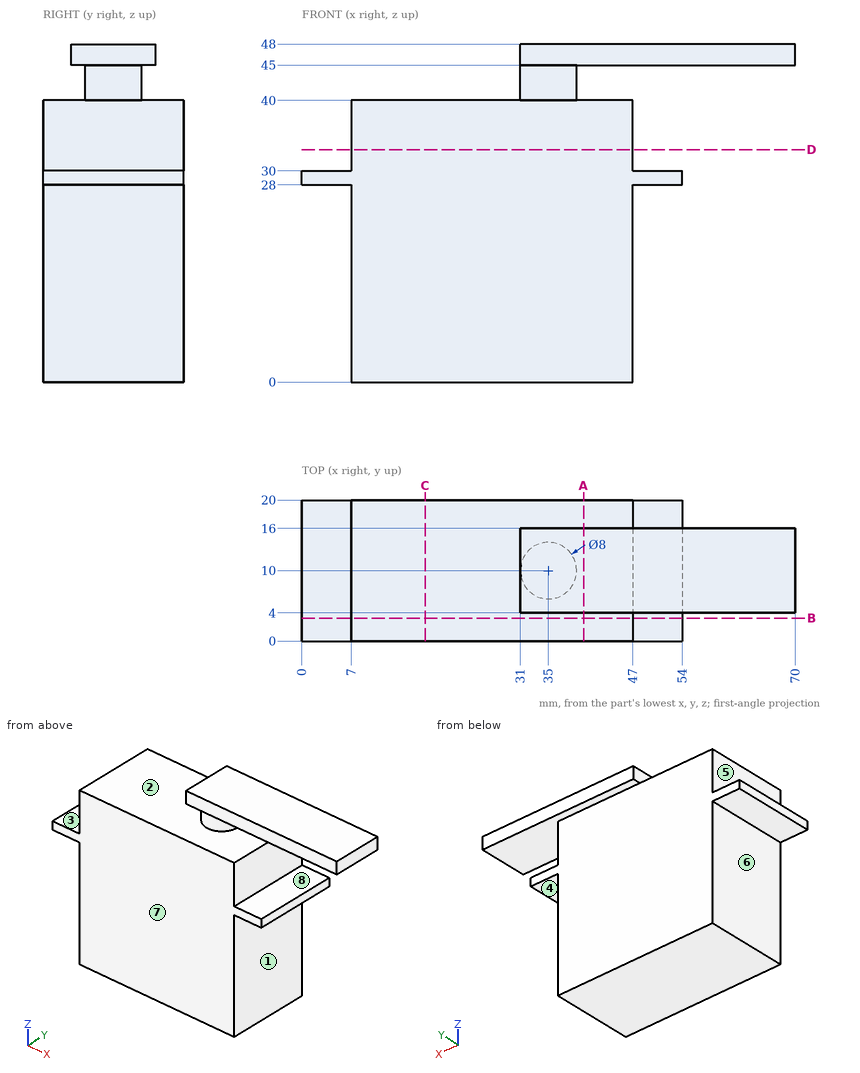
The drawing under review shows one solid part. Ordinate dimensions are in mm from its lowest x, y, z. A direction names the side the tool comes from. Give positions to 0.01 mm unless a question says otherwise; leave off trailing zeros. Loops run counter-clockwise (first coordinate to the right, second up) from the corner with the lowest first, then second, coordinate; pieces in that order, holes last. Notation, with made-up numbers: M -8.75,-2.5 L 50.25,-2.5 A25 cw 50.25,35.5 Z; hole C 86.5,88.5 d8. An arc over 180 degrees is marked long. One line per item, written item: value. Start each with the question number.
Q1. Clearance check with flat-ended pins moving along their axes: pin 1 Ø10 at (y, z) = (13.5, 17) entering from +X; pin 2 Ø3.5 at (y, z) = (9, 47) entering from -X; pin 3 Ø5 at (y, z) = (6.5, 34.5) entering from -X. State where each tip first meets the part, or that it passes through.
Q2. Machinability: for the marked faces 4, 5, 6, 7 and 8, which of the approach directions +Z, -Z, +X, -X, +Y, -Y give a long, thin tool a straight path to every point of the face, cutting with its end or side? Answer none if there is none.
Q3. Draft analysis for pull direction Z (two halves, no side actions). For the marked faces 1, 2 and 3, state which applies: released by +Z, released by -Z, zero draft, split by the parting line, or undercut.
Q4. Add section B-B (y = 3.25). Give the boundary of the cut face in (x, z).
Q5. Add section C-C (x = 17.5). Give the boundary of the cut face in (y, z), and give its area (3 significant figures).
Q6. Add section D-D (z = 33). Give the boundary of the cut face in (x, y), and give its area (3 significant figures).
Q7. Add section A-A (x = 40). Give the boundary of the cut face in (y, z).
Q8. For L1, parallel to Z at x = 40.5, y = 5; L2, parallel to Z at x = 51, y = 2.25; L3, parallel to X at y = 12, z = 34.5, list the stretches that pass through material, from the lowest coordinate up.
Reply:
1. pin 1: x = 47
1. pin 2: x = 31
1. pin 3: x = 7
2. face 4: -Z, +X, +Y, -Y
2. face 5: +Z, -X, +Y, -Y
2. face 6: -Z, -X, +Y, -Y
2. face 7: +Z, -Z, +X, -X, -Y
2. face 8: +X, +Y, -Y
3. face 1: zero draft
3. face 2: undercut
3. face 3: released by +Z
4. outline: M 0,28 L 7,28 L 7,0 L 47,0 L 47,28 L 54,28 L 54,30 L 47,30 L 47,40 L 7,40 L 7,30 L 0,30 Z
5. outline: M 0,0 L 20,0 L 20,40 L 0,40 Z
5. area: 800 mm²
6. outline: M 7,0 L 47,0 L 47,20 L 7,20 Z
6. area: 800 mm²
7. outline: M 0,0 L 20,0 L 20,40 L 0,40 Z; M 4,45 L 16,45 L 16,48 L 4,48 Z
8. L1: 0 to 40, 45 to 48
8. L2: 28 to 30
8. L3: 7 to 47
